Design review of the part built by this model. Coordinates are the model's own, in mm. Face numbers are marked on the shaded views. A direction names the side the tool comes from. Coordinates: 2 decimals unless noted, no trailing zeros. Order: outer loops, then holes, each group sorted by start corner. A loop starts at its lowest first (then second) coordinate and runs counter-clockwise, first axis right, second up.
from build123d import *

# Parameters (mm, degrees)
SKETCH1_R           = 50
BOSS_EXTRUDE1_DEPTH = 30
SKETCH2_W           = 10
SKETCH2_H           = 50
BOSS_EXTRUDE2_DEPTH = 50
CUT_EXTRUDE2_DEPTH  = 50
SKETCH5_R           = 7.5
CUT_EXTRUDE3_DEPTH  = 50


with BuildPart() as part:
    # Sketch1 → Boss-Extrude1 (new body)
    with BuildSketch(Plane(origin=(0, 0, 0), x_dir=(1, 0, 0), z_dir=(0, 1, 0))):
        Circle(SKETCH1_R)
    extrude(amount=BOSS_EXTRUDE1_DEPTH)

    # Sketch2 → Boss-Extrude2 (add)
    with BuildSketch(Plane(origin=(0, 30, 0), x_dir=(1, 0, 0), z_dir=(0, 1, 0))):
        with Locations((-20, 0)):
            Rectangle(SKETCH2_W, SKETCH2_H)
        with Locations((20, 0)):
            Rectangle(SKETCH2_W, SKETCH2_H)
    extrude(amount=BOSS_EXTRUDE2_DEPTH)

    # Sketch4 → Cut-Extrude2 (cut)
    with BuildSketch(Plane.ZY.offset(25)):
        with BuildLine():
            Line((30.852726851, 88.254535322), (30.852726851, 55))
            Line((30.852726851, 55), (25, 55))
            ThreePointArc((25, 55), (0, 80), (-25, 55))
            Line((-25, 55), (-34.201839493, 55))
            Line((-34.201839493, 55), (-34.201839493, 88.254535322))
            Line((-34.201839493, 88.254535322), (30.852726851, 88.254535322))
        make_face()
    extrude(amount=-CUT_EXTRUDE2_DEPTH, mode=Mode.SUBTRACT)

    # Sketch5 → Cut-Extrude3 (cut)
    with BuildSketch(Plane.ZY.offset(25)):
        with Locations((0, 55)):
            Circle(SKETCH5_R)
    extrude(amount=-CUT_EXTRUDE3_DEPTH, mode=Mode.SUBTRACT)


solid = part.part
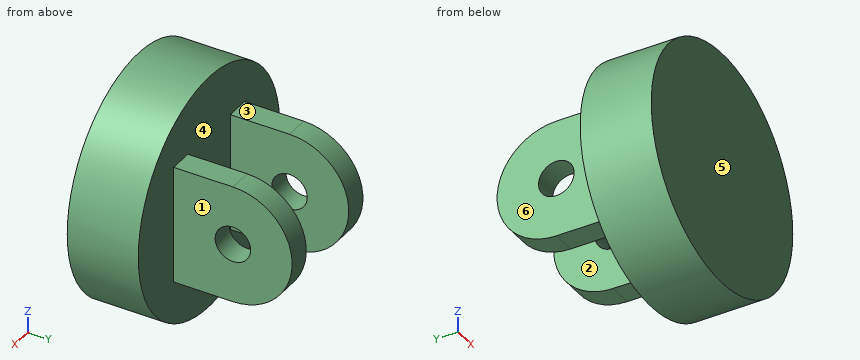
1. Add section D-D (x = 0). Give the boundary of the cut face in (y, z), and give its area (3 significant figures).
2. For the marked faces 1, 2 and 3, list the 3-axis set-ups (+Z, -Z, +X, -X, +Y, -Y) from which the entire face can be reached by the end or side of a thin tool; tool diameter is ignored.
3. Insertion check: pin 1 (3 mm diameter, centred on x = -18.5, y = 43, fed in from -Z); pin 2 (3 mm diameter, centred on x = 21, y = 41.5, fed in from +Z); pin 3 (1 mm diameter, centred on y = 35, z = 4, fed in from +X). Each pin has a flat end and moves straight along its axis. Give the tip position at first contact, or say it passes through.
4. Add section A-A (y = 73). Give the boundary of the cut face in (x, z), and give its area (3 significant figures).
5. Add section C-C (z = 4). Give the boundary of the cut face in (x, y).
6. Mouldability with a two-part tool opening along X and no side actions: class the marked faces 4, 5 and 6 as pulls with the +X half, pulls with the -X half, needs draft (parallel to the pull), parting line crosses it, or undercut.
7. Add section B-B (x = 22.5). Give the boundary of the cut face in (y, z), and give its area (3 significant figures).
8. To check wall thickness, follow line 1 (Y direction, x = -19, z = 0); line 2 (X direction, y = 64.5, z = 8.5); line 3 (Y direction, x = 44, z = -13). State the ranges of each line that lie inside material, in increasing order.
Solution:
1. outline: (0, -50) - (30, -50) - (30, 50) - (0, 50) - close
1. area: 3,000 mm2
2. face 1: +Z, -Z, +X, +Y
2. face 2: +Z, -Z, +Y
2. face 3: +Z, +X, -X, +Y
3. pin 1: stops at z = -25
3. pin 2: stops at z = 25
3. pin 3: stops at x = 25
4. outline: (-25, -17.35) - (-15, -17.35) - (-15, 17.35) - (-25, 17.35) - close; (15, -17.35) - (25, -17.35) - (25, 17.35) - (15, 17.35) - close
4. area: 694 mm2
5. outline: (-49.84, 0) - (49.84, 0) - (49.84, 30) - (25, 30) - (25, 48.66) - (15, 48.66) - (15, 30) - (-15, 30) - (-15, 48.66) - (-25, 48.66) - (-25, 30) - (-49.84, 30) - close; (-25, 61.34) - (-15, 61.34) - (-15, 79.68) - (-25, 79.68) - close; (15, 61.34) - (25, 61.34) - (25, 79.68) - (15, 79.68) - close
6. face 4: undercut
6. face 5: needs draft
6. face 6: pulls with the -X half
7. outline: (0, -44.65) - (30, -44.65) - (30, -25) - (55, -25) arc R25 ccw to (55, 25) - (30, 25) - (30, 44.65) - (0, 44.65) - close; hole circle Ø15 at (55, 0)
7. area: 4,730 mm2
8. line 1: y = 0 to 47.5, 62.5 to 80
8. line 2: x = -25 to -15, 15 to 25
8. line 3: y = 0 to 30
